Autodesk Fusion 360 part; units mm, degrees
sketch "Sketch1" plane through (0, 0, 0) normal (1, 0, 0) x (0, 0, -1)
  line L0 (0, 0) -> (0, 37)
  line L1 (0, 37) -> (-20, 37)
  line L2 (-20, 37) -> (-20, 40)
  line L3 (-20, 40) -> (40, 40)
  line L4 (40, 40) -> (40, 37)
  line L5 (40, 37) -> (20, 37)
  line L6 (20, 37) -> (20, 0)
  line L7 (20, 0) -> (0, 0)
  line L8 (0, 4.5) -> (20, 4.5)
  line L9 (20, 4.5) -> (20, 7.5)
  line L10 (20, 7.5) -> (0, 7.5)
  line L11 (0, 7.5) -> (0, 4.5)
  line L12 (10, 0) -> (10, 40) construction
  point P0 (10, 40)
  dimension "d1" = 20
  dimension "d2" = 4.5
  dimension "d3" = 3
  dimension "d5" = 40
  dimension "d7" = 3
  dimension "d8" = 60
extrude "Extrude1" add sketch "Sketch1" along normal blind 4 makes body 1
extrude "Extrude2" add sketch "Sketch1" along normal blind 11 separate body contours L0 L6 L8 L9 L10 L11 makes body 2
sketch "Sketch2" plane through (0, 7.5, 0) normal (0, 1, 0) x (-1, 0, 0)
  line L0 (0, -20) -> (0, 0)
  line L1 (0, 0) -> (-11, 0)
  line L2 (-11, 0) -> (-11, -20)
  line L3 (-11, -20) -> (0, -20)
  circle A0 centre (-8.35, -17.25) radius 1.65
  circle A1 centre (-8.35, -2.75) radius 1.65
  line L4 (-8.35, -2.75) -> (-8.35, -17.25) construction
  line L5 (-11, -10) -> (-5.7, -10) construction
  point P0 (-8.35, -10)
  dimension "d15" = 14.5
  dimension "d16" = 2.65
  dimension "d17" = 3.3
  dimension "d18" = 3.3
extrude "Extrude3" cut sketch "Sketch2" against normal through all contours A0 | A1 bodies 2
sketch "Sketch3" plane through (0, 40, 0) normal (0, 1, 0) x (-1, 0, 0)
  line L0 (0, -40) -> (0, 20)
  line L1 (0, 20) -> (-4, 20)
  line L2 (-4, 20) -> (-4, -40)
  line L3 (-4, -40) -> (0, -40)
sketch "Sketch4" plane through (0, 40, 0) normal (0, 1, 0) x (-1, 0, 0)
  circle A0 centre (-15.35, -30) radius 1.65
  circle A1 centre (-15.35, 10) radius 1.65
  line L0 (-15.35, 10) -> (-15.35, -30) construction
  line L1 (0, 20) -> (0, -40)
  line L2 (0, -10) -> (-15.35, -10) construction
  dimension "d20" = 40
  dimension "d21" = 3.3
  dimension "d22" = 3.3
  dimension "d23" = 15.35
sketch "Sketch5" plane through (4, 0, 0) normal (1, 0, 0) x (0, 0, -1)
  line L0 (0, 37) -> (0, 0)
  line L1 (0, 0) -> (20, 0)
  line L2 (20, 0) -> (20, 37)
  line L3 (20, 37) -> (40, 37)
  line L4 (40, 37) -> (40, 40)
  line L5 (40, 40) -> (-20, 40)
  line L6 (-20, 40) -> (-20, 37)
  line L7 (-20, 37) -> (0, 37)
  line L8 (-14, 40) -> (-6, 40)
  line L9 (-6, 40) -> (-6, 37)
  line L10 (-6, 37) -> (-14, 37)
  line L11 (-14, 37) -> (-14, 40)
  line L12 (26, 40) -> (34, 40)
  line L13 (34, 40) -> (34, 37)
  line L14 (34, 37) -> (26, 37)
  line L15 (26, 37) -> (26, 40)
  point P0 (-10, 40)
  point P1 (30, 40)
  dimension "d24" = 8
  dimension "d25" = 8
  dimension "d26" = 4
  dimension "d27" = 4
extrude "Extrude4" add sketch "Sketch5" along normal blind 15 contours L5 L7 L8 L9 L10 L11 | L3 L5 L12 L13 L14 L15 bodies 1
extrude "Extrude5" cut sketch "Sketch4" against normal through all bodies 1
combine "Combine1" operation add target body 2 tool bodies 1
equation "d3 = Linear Dimension-4"
equation "d7 = Linear Dimension-6"
equation "d16 = 1 mm + ( 3.3 / 2 ) * 1 mm"
equation "d17 = Diameter Dimension-2"
equation "d18 = Diameter Dimension-3"
equation "d21 = Diameter Dimension-2"
equation "d22 = Diameter Dimension-3"
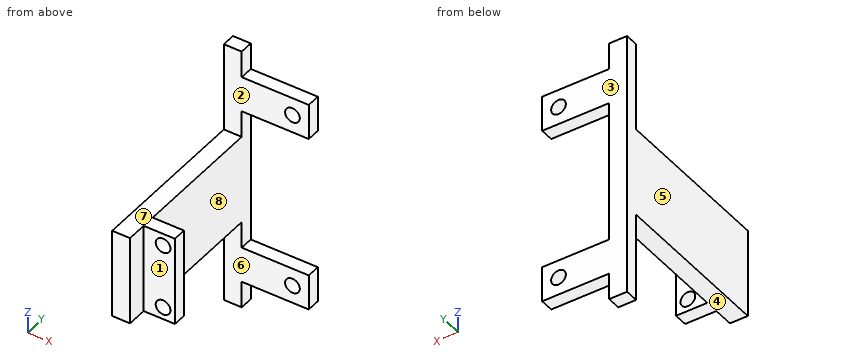
Geometry: final body of the model. Coordinates: model frame, mm. Face numbers are marked on the shaded views. A direction names the side the tool comes from. Coordinates: 2 decimals unless noted, no trailing zeros. Order: outer loops, then holes, each group sorted by start corner. A loop starts at its lowest first (then second) coordinate and runs counter-clockwise, first axis right, second up. Notation, with made-up numbers: (25, 22.5) - (83, 22.5) arc R33 ccw to (83, 51.5) - close; hole circle Ø8 at (30.25, 16.5). An arc over 180 degrees is marked (long way). Write each question's results on one line, items separated by ' | '.
(1) Section query C-C, the plane x = 8.35. Return the cut outline in (y, z), plus the area to 3 significant figures.
Values found:
outline: (4.5, -20) - (7.5, -20) - (7.5, -18.9) - (4.5, -18.9) - close; (4.5, -15.6) - (7.5, -15.6) - (7.5, -4.4) - (4.5, -4.4) - close; (4.5, -1.1) - (7.5, -1.1) - (7.5, 0) - (4.5, 0) - close; (37, -34) - (40, -34) - (40, -26) - (37, -26) - close; (37, 6) - (40, 6) - (40, 14) - (37, 14) - close | area: 88.2 mm²
(2) Set-up query: the marked faces 1, 2, 3, 4 and 5. Return all of +Z, -Z, +X, -X, +Y, -Y with unobstructed straight access to the full face (end or side cutting, diameter ignored); none if empty.
Values found:
face 1: +Z, -Z, +X, -Y | face 2: +Z, +X, -X, -Y | face 3: +Z, -Z, +X, -X, +Y | face 4: -Z, +X, -X, -Y | face 5: +Z, -Z, -X, +Y, -Y
(3) Section query A-A, the plane z = -2.75. Return the cut outline in (x, y), plus the area to 3 significant figures.
Values found:
outline: (0, 0) - (4, 0) - (4, 4.5) - (6.7, 4.5) - (6.7, 7.5) - (4, 7.5) - (4, 40) - (0, 40) - close; (10, 4.5) - (11, 4.5) - (11, 7.5) - (10, 7.5) - close | area: 171 mm²
(4) First-contact query: pin 1 Ø0.9 at (y, z) = (38, -38) entering from +X; pin 2 Ø0.9 at (y, z) = (6.5, -10.5) entering from +X; pin 3 Ø2 at (y, z) = (18.5, -22) entering from -X; pin 4 Ø2 at (x, z) = (10, 10) entering from -Y. Flat tips, straight axial feed; report the tip coordinate or a pass-through.
Values found:
pin 1: stops at x = 4 | pin 2: stops at x = 11 | pin 3: passes through | pin 4: stops at y = 37
(5) Line query: line 1 (Z direction, x = 8.35, y = 6.3); line 2 (Z direction, x = 15.35, y = 38.2); line 3 (Y direction, x = 6.5, z = -2). Output: solid intervals per line, ascending. Write a range as [from, to].
Values found:
line 1: z = [-20, -18.9], [-15.6, -4.4], [-1.1, 0] | line 2: z = [-34, -31.65], [-28.35, -26], [6, 8.35], [11.65, 14] | line 3: y = [4.5, 7.5]
(6) Mould query, pull axis Z, two halves, no side actions, for the marked faces 6, 7 and 8. Classes: +Z half, -Z half, draft (parallel to the pull), parting line (faces both ways), or undercut.
Values found:
face 6: draft | face 7: +Z half | face 8: undercut
(7) Section query D-D, the plane x = 15.35. Return the cut outline in (y, z), plus the area to 3 significant figures.
Values found:
outline: (37, -34) - (40, -34) - (40, -31.65) - (37, -31.65) - close; (37, -28.35) - (40, -28.35) - (40, -26) - (37, -26) - close; (37, 6) - (40, 6) - (40, 8.35) - (37, 8.35) - close; (37, 11.65) - (40, 11.65) - (40, 14) - (37, 14) - close | area: 28.2 mm²
(8) Section query B-B, the plane x = 4.75. Return the cut outline in (y, z), plus the area to 3 significant figures.
Values found:
outline: (4.5, -20) - (7.5, -20) - (7.5, 0) - (4.5, 0) - close; (37, -34) - (40, -34) - (40, -26) - (37, -26) - close; (37, 6) - (40, 6) - (40, 14) - (37, 14) - close | area: 108 mm²
